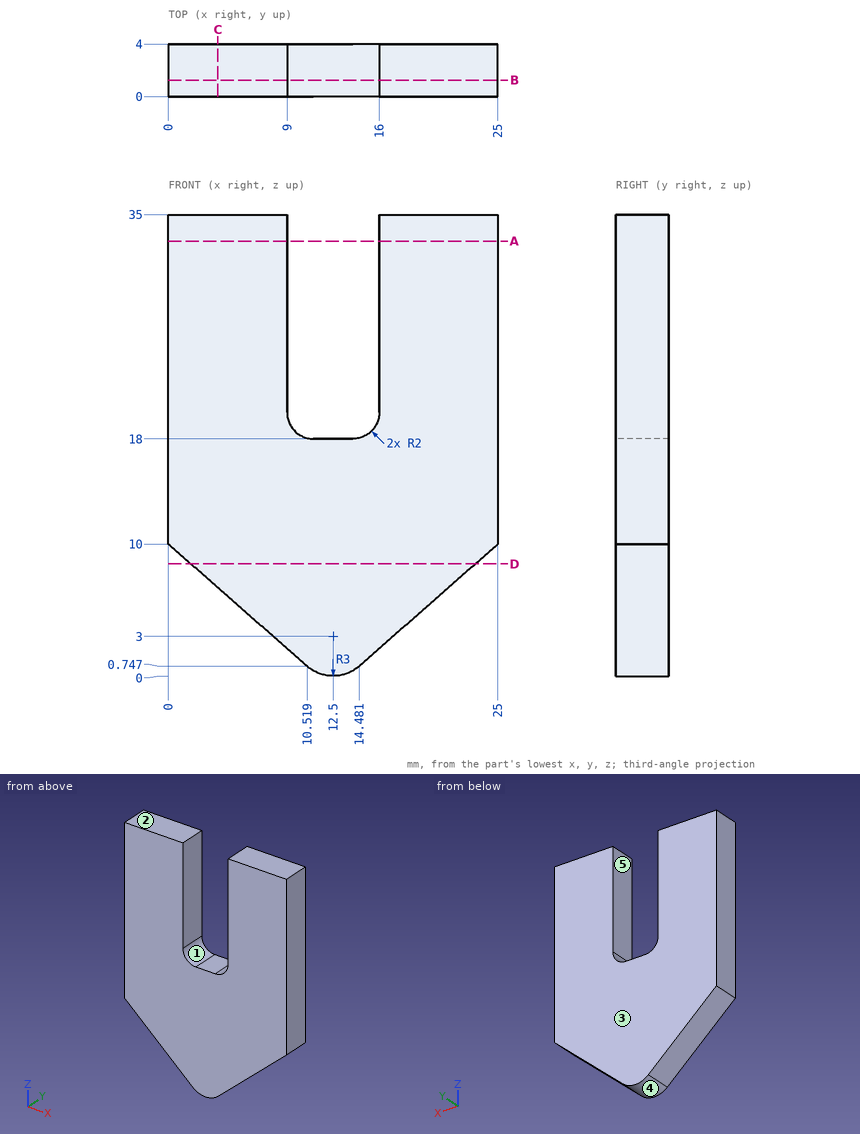
Here's the drawing with two shaded views (mm, measured from the low corner). I have some questions. A direction names the side the tool comes from. Give positions to 0.01 mm unless a question says otherwise; leave off trailing zeros. Loops run counter-clockwise (first coordinate to the right, second up) from the corner with the lowest first, then second, coordinate; pieces in that order, holes last. Notation, with made-up numbers: (82.5, 28) - (119.5, 28) arc R28 cw to (119.5, 58) - close; hole circle Ø9 at (10.25, 14.25). An arc over 180 degrees is marked (long way). Answer in a Markdown table with one row per item. Add a question column.
Q1. If we section it at B-B (y = 1.25): List the corners of the cut face in (x, z) for me, plus the area to 3 significant figures.
Q2. Please list where these lines run through material, in increasing order: L1, parallel to X at y = 2, z = 30.5; L2, parallel to X at y = 3.4, z = 9 (1 decimal); L3, parallel to Z at x = 4.25, y = 2.8. Write a range as from..to.
Q3. We'd pull the mould along X, two halves only. Please class the marked faces 3, 4 and 5: +X half, -X half, draft (parallel to the pull), parting line (faces both ways), or undercut.
Q4. For pin 1 (0.9 mm diameter, centred on x = 12.5, y = 2.5, fed in from +Z), with a flat end and sliding along its axis, tell me the tip position at first contact or that it passes through.
Q5. If we section it at C-C (x = 3.75): List the corners of the cut face in (y, z) for me, plus the area to 3 significant figures.
Q6. Which directions (+Z, -Z, +X, -X, +Y, -Y) give clear straight access to the entire face, cutting with the end or side of a thin tool? Please do the marked faces 1 and 2.
Q7. If we section it at D-D (z = 8.5): List the corners of the cut face in (x, y) for me (1 decimal).
Q8. If we section it at A-A (z = 33): List the corners of the cut face in (x, y) for me.
The answers:
| question | item | result |
|---|---|---|
| 1 | outline | (0, 10) - (10.52, 0.75) arc R3 ccw to (14.48, 0.75) - (25, 10) - (25, 35) - (16, 35) - (16, 20) arc R2 cw to (14, 18) - (11, 18) arc R2 cw to (9, 20) - (9, 35) - (0, 35) - close |
| 1 | area | 644 mm^2 |
| 2 | L1 | x = 0..9, 16..25 |
| 2 | L2 | x = 1.1..23.9 |
| 2 | L3 | z = 6.26..35 |
| 3 | face 3 | draft |
| 3 | face 4 | parting line |
| 3 | face 5 | undercut |
| 4 | pin 1 | stops at z = 18 |
| 5 | outline | (0, 6.7) - (4, 6.7) - (4, 35) - (0, 35) - close |
| 5 | area | 113 mm^2 |
| 6 | face 1 | +Z, +Y, -Y |
| 6 | face 2 | +Z, +X, -X, +Y, -Y |
| 7 | outline | (1.7, 0) - (23.3, 0) - (23.3, 4) - (1.7, 4) - close |
| 8 | outline | (0, 0) - (9, 0) - (9, 4) - (0, 4) - close; (16, 0) - (25, 0) - (25, 4) - (16, 4) - close |
